Verification items for the finished model (mm, model axes). A direction names the side the tool comes from. Coordinates: 2 decimals unless noted, no trailing zeros. Loops run counter-clockwise (first coordinate to the right, second up) from the corner with the lowest first, then second, coordinate; pieces in that order, holes last. Notation, with made-up numbers: (2, -10) -> (54, -10) arc R31 ccw to (54, 20) -> close; hole circle Ø6 at (85.25, 1.25). An arc over 180 degrees is marked (long way). Answer as a JSON object with one key per item and string values. Group by question number.
Q1. Release check for a two-part mould opening along Y. For faces 6 (the flat face through (-42.78, 6.439, 1.096)), 7 (the cylindrical face through (42.455, 3.164, -3.751)), 8 (the flat face through (62.5, 3, -3)), 9 (the flat face through (-35, 0, 1)) record: released by +Y, released by -Y, zero draft, split by the parting line, or undercut.
Q2. Cross-section at A-A on x = 0. Record the boundary of the cut face in (y, z), and give its area (3 significant figures).
Q3. Cross-section at B-B on x = 31. Record the boundary of the cut face in (y, z), and give its area (3 significant figures).
Q4. Set-up check for faces 1 (the conical face through (-2.94, 10.51, 0.65)), 2 (the flat face through (-6.35, 3, 0)), 3 (the flat face through (-22.5, 8, -1)), 4 (the flat face through (42.78, 6.439, -1.096)), 5 (the flat face through (34, 0, 0)): record each of +Z, -Z, +X, -X, +Y, -Y from which the full face is reachable in a straight line by a thin tool's end or side.
Q5. Scan lines: L1, parallel to Z at x = 0, y = 7.55; L2, parallel to X at y = 7.3, z = 0; L3, parallel to X at y = 2.5, z = 2. Record each from-to range of solid material in increasing order.
Q6. Gauge pin test, flat ends, axial feed: pin 1 Ø1 at (x, z) = (-30.5, -2.5) entering from +Y; pin 2 Ø6.5 at (x, z) = (0, 0) entering from +Y; pin 3 Ø3 at (y, z) = (6, -2.5) entering from -X. Record the tip position at first contact, or that the pin passes through.
```python
from build123d import *

# Parameters (mm, degrees)
SKETCH1_W                                       = 125
SKETCH1_H                                       = 12.7
BOSS_EXTRUDE1_DEPTH                             = 12.7
SKETCH2_W                                       = 12.7
SKETCH2_H                                       = 12.7
CUT_EXTRUDE1_DEPTH                              = 6.35
CSK_FOR_M5_FLAT_HEAD_MACHINE_SCREW1_D           = 5.8
CSK_FOR_M5_FLAT_HEAD_MACHINE_SCREW1_CSINK_D     = 10.4
CSK_FOR_M5_FLAT_HEAD_MACHINE_SCREW1_CSINK_ANGLE = 90
CUT_EXTRUDE2_DEPTH                              = 40
TAP_DRILL_FOR_M2_5X0_45_TAP1_D                  = 2.05
TAP_DRILL_FOR_M2_5X0_45_TAP1_DEPTH              = 8.164811475
CIRPATTERN1_COUNT                               = 2


with BuildPart() as part:
    # Sketch1 → Boss-Extrude1 (new body)
    with BuildSketch(Plane(origin=(0, 0, 0), x_dir=(1, 0, 0), z_dir=(0, 1, 0))):
        Rectangle(SKETCH1_W, SKETCH1_H)
    extrude(amount=BOSS_EXTRUDE1_DEPTH)

    # Sketch2 → Cut-Extrude1 (cut)
    with BuildSketch(Plane.XZ):
        Rectangle(SKETCH2_W, SKETCH2_H)
    extrude(amount=-CUT_EXTRUDE1_DEPTH, mode=Mode.SUBTRACT)

    # CSK for M5 Flat Head Machine Screw1 (through all)
    with Locations(Plane.ZX.offset(12.7)):
        with Locations((0, 0)):
            CounterSinkHole(CSK_FOR_M5_FLAT_HEAD_MACHINE_SCREW1_D / 2, CSK_FOR_M5_FLAT_HEAD_MACHINE_SCREW1_CSINK_D / 2, counter_sink_angle=CSK_FOR_M5_FLAT_HEAD_MACHINE_SCREW1_CSINK_ANGLE)

    # Sketch7 → Cut-Extrude2 (cut)
    with BuildSketch(Plane(origin=(62.5, 0, 0), x_dir=(0, 0, -1), z_dir=(1, 0, 0))):
        Polygon((6.35, 12.7), (-6.35, -2.435270626), (-6.35, 12.7), align=None)
    cut_extrude2 = extrude(amount=-CUT_EXTRUDE2_DEPTH, mode=Mode.SUBTRACT)

    # Tap Drill for M2.5x0.45 Tap1
    with Locations(Plane(origin=(42.5, 5.039555569, 0.077876097), x_dir=(0, 0.766044443119, -0.642787609687), z_dir=(0, 0.642787609687, 0.766044443119))):
        with Locations((0, 0)):
            tap_drill_for_m2_5x0_45_tap1 = Hole(TAP_DRILL_FOR_M2_5X0_45_TAP1_D / 2, depth=TAP_DRILL_FOR_M2_5X0_45_TAP1_DEPTH)

    # CirPattern1: Cut-Extrude2, Tap Drill for M2.5x0.45 Tap1 ×2 about axis
    cirpattern1_axis = Axis((0, 0, 0), (0, 1, 0))
    add([cut_extrude2.rotate(cirpattern1_axis, i * 360 / CIRPATTERN1_COUNT) for i in range(1, CIRPATTERN1_COUNT)], mode=Mode.SUBTRACT)
    add([tap_drill_for_m2_5x0_45_tap1.rotate(cirpattern1_axis, i * 360 / CIRPATTERN1_COUNT) for i in range(1, CIRPATTERN1_COUNT)], mode=Mode.SUBTRACT)


solid = part.part
```
Computed values:
{
 "1": {"face 6": "released by +Y", "face 7": "undercut", "face 8": "zero draft", "face 9": "released by -Y"},
 "2": {"outline": "(6.35, -6.35) -> (12.7, -6.35) -> (12.7, -5.2) -> (10.4, -2.9) -> (6.35, -2.9) -> close; (6.35, 2.9) -> (10.4, 2.9) -> (12.7, 5.2) -> (12.7, 6.35) -> (6.35, 6.35) -> close", "area": "38.5 mm²"},
 "3": {"outline": "(0, -6.35) -> (12.7, -6.35) -> (0, 4.31) -> close", "area": "67.7 mm²"},
 "4": {"face 1": "+Y", "face 2": "+Z, -Z, -Y", "face 3": "-Z, -X, +Y", "face 4": "+Z, +X, +Y", "face 5": "+Z, -Z, +X, -X, -Y"},
 "5": {"L1": "z = -6.35 to -2.9, 2.9 to 6.35", "L2": "x = -22.5 to -2.9, 2.9 to 22.5", "L3": "x = -62.5 to -43.32, -41.68 to -6.35, 6.35 to 62.5"},
 "6": {"pin 1": "stops at y = 2.75", "pin 2": "stops at y = 10.75", "pin 3": "stops at x = -22.5"}
}
